Part model, mm, in its own coordinate system. A direction names the side the tool comes from. Round coordinates to 2 decimals unless told otherwise and drop trailing zeros. Write each loop counter-clockwise with the first axis right and the second up, starting at its lowest first coordinate (ties: lowest second). Pieces come first, ordered by that corner, then holes.
```python
from build123d import *

# Parameters (mm, degrees)
F0_W     = 25.4
F0_H     = 25.4
F0_W_2   = 23.368
F0_H_2   = 23.368
F1_DEPTH = 711.2
F2_R     = 2.1844
F3_DEPTH = 25.4
F4_R     = 2.1844
F5_DEPTH = 25.4


with BuildPart() as f1:
    # F0 (on Top) → F1 (new body)
    with BuildSketch(Plane.XY):
        with Locations((12.7, -12.7)):
            Rectangle(F0_W, F0_H)
        with Locations((12.7, -12.7)):
            Rectangle(F0_W_2, F0_H_2, mode=Mode.SUBTRACT)
    extrude(amount=F1_DEPTH)

    # F2 (on face) → F3 (cut)
    with BuildSketch(Plane.XZ.offset(25.4)):
        with Locations((12.7, 12.7)):
            Circle(F2_R)
        with Locations((12.7, 38.1)):
            Circle(F2_R)
        with Locations((12.7, 241.3)):
            Circle(F2_R)
        with Locations((12.7, 215.9)):
            Circle(F2_R)
        with Locations((12.7, 190.5)):
            Circle(F2_R)
        with Locations((12.7, 165.1)):
            Circle(F2_R)
        with Locations((12.7, 139.7)):
            Circle(F2_R)
        with Locations((12.7, 114.3)):
            Circle(F2_R)
        with Locations((12.7, 88.9)):
            Circle(F2_R)
        with Locations((12.7, 63.5)):
            Circle(F2_R)
        with Locations((12.7, 266.7)):
            Circle(F2_R)
        with Locations((12.7, 292.1)):
            Circle(F2_R)
        with Locations((12.7, 317.5)):
            Circle(F2_R)
        with Locations((12.7, 342.9)):
            Circle(F2_R)
        with Locations((12.7, 368.3)):
            Circle(F2_R)
        with Locations((12.7, 393.7)):
            Circle(F2_R)
        with Locations((12.7, 419.1)):
            Circle(F2_R)
        with Locations((12.7, 444.5)):
            Circle(F2_R)
        with Locations((12.7, 469.9)):
            Circle(F2_R)
        with Locations((12.7, 495.3)):
            Circle(F2_R)
        with Locations((12.7, 520.7)):
            Circle(F2_R)
        with Locations((12.7, 546.1)):
            Circle(F2_R)
        with Locations((12.7, 571.5)):
            Circle(F2_R)
        with Locations((12.7, 596.9)):
            Circle(F2_R)
        with Locations((12.7, 622.3)):
            Circle(F2_R)
        with Locations((12.7, 647.7)):
            Circle(F2_R)
        with Locations((12.7, 673.1)):
            Circle(F2_R)
        with Locations((12.7, 698.5)):
            Circle(F2_R)
    extrude(amount=-F3_DEPTH, mode=Mode.SUBTRACT)

    # F4 (on face) → F5 (cut)
    with BuildSketch(Plane(origin=(0, 0, 0), x_dir=(0, -1, 0), z_dir=(-1, 0, 0))):
        with Locations((12.7, 12.7)):
            Circle(F4_R)
        with Locations((12.7, 38.1)):
            Circle(F4_R)
        with Locations((12.7, 63.5)):
            Circle(F4_R)
        with Locations((12.7, 88.9)):
            Circle(F4_R)
        with Locations((12.7, 114.3)):
            Circle(F4_R)
        with Locations((12.7, 139.7)):
            Circle(F4_R)
        with Locations((12.7, 165.1)):
            Circle(F4_R)
        with Locations((12.7, 190.5)):
            Circle(F4_R)
        with Locations((12.7, 215.9)):
            Circle(F4_R)
        with Locations((12.7, 241.3)):
            Circle(F4_R)
        with Locations((12.7, 266.7)):
            Circle(F4_R)
        with Locations((12.7, 292.1)):
            Circle(F4_R)
        with Locations((12.7, 317.5)):
            Circle(F4_R)
        with Locations((12.7, 342.9)):
            Circle(F4_R)
        with Locations((12.7, 368.3)):
            Circle(F4_R)
        with Locations((12.7, 393.7)):
            Circle(F4_R)
        with Locations((12.7, 419.1)):
            Circle(F4_R)
        with Locations((12.7, 444.5)):
            Circle(F4_R)
        with Locations((12.7, 546.1)):
            Circle(F4_R)
        with Locations((12.7, 520.7)):
            Circle(F4_R)
        with Locations((12.7, 495.3)):
            Circle(F4_R)
        with Locations((12.7, 469.9)):
            Circle(F4_R)
        with Locations((12.7, 571.5)):
            Circle(F4_R)
        with Locations((12.7, 596.9)):
            Circle(F4_R)
        with Locations((12.7, 622.3)):
            Circle(F4_R)
        with Locations((12.7, 647.7)):
            Circle(F4_R)
        with Locations((12.7, 673.1)):
            Circle(F4_R)
        with Locations((12.7, 698.5)):
            Circle(F4_R)
    extrude(amount=-F5_DEPTH, mode=Mode.SUBTRACT)


solid = f1.part
```
Q1. Wall check: L1, parallel to Y at x = 13, z = 202.5; L2, parallel to X at y = -8.25, z = 172.5; L3, parallel to X at y = -25.05, z = 444.5. Give the ranges that are in metal, low to high.
Values follow:
L1: y = -25.4 to -24.38, -1.02 to 0
L2: x = 0 to 1.02, 24.38 to 25.4
L3: x = 0 to 10.52, 14.88 to 25.4
Q2. Cut at A-A on y = -5. Write the cut outline in (x, z).
Values follow:
outline: (0, 0) - (1.02, 0) - (1.02, 711.2) - (0, 711.2) - close; (24.38, 0) - (25.4, 0) - (25.4, 711.2) - (24.38, 711.2) - close
Q3. Cut at B-B on z = 409.5. Write the cut outline in (x, y), plus the area to 3 significant figures.
Values follow:
outline: (0, -25.4) - (25.4, -25.4) - (25.4, 0) - (0, 0) - close; hole (1.02, -24.38) - (24.38, -24.38) - (24.38, -1.02) - (1.02, -1.02) - close
area: 99.1 mm2
Q4. Drop a flat-ended pin along its axis: pin 1 (4 mm diameter, centred on x = 12.7, z = 266.7, fed in from -Y). Give the stop position or say it passes through.
Values follow:
pin 1: passes through
Q5. Which spindle directions (+Z, -Z, +X, -X, +Y, -Y) get a long thin tool onto all of the face, cutting with end or side? Do faces 1 (the flat face through (13, -1.016, 351)), 2 (the flat face through (0, -13, 351)). Say none if no direction does.
Values follow:
face 1: +Z, -Z
face 2: +Z, -Z, -X, +Y, -Y
Q6. Mould opens along Y. For faces 3 (the flat face through (25.4, -13, 351)), 4 (the flat face through (24.384, -13, 351)), 5 (the flat face through (13, -25.4, 351)), 6 (the flat face through (13, -24.384, 351)) say: +Y half, -Y half, draft (parallel to the pull), parting line (faces both ways), or undercut.
Values follow:
face 3: draft
face 4: undercut
face 5: -Y half
face 6: undercut
